Answer from the drawing. Dimensions are ordinates in mm from the lowest x, y and z of the part. A direction names the side the tool comes from. Coordinates: 2 decimals unless noted, no trailing zeros. Loops run counter-clockwise (first coordinate to the right, second up) from the corner with the lowest first, then second, coordinate; pieces in that order, holes last. Notation, with made-up numbers: (33.25, 54.25) - (88.25, 54.25) arc R15 cw to (88.25, 74.25) - close; hole circle Ø3 at (79, 74.25). An arc over 180 degrees is marked (long way). Use one line per item in the form item = value. Start each with the question number.
1) A cutting plane is placed at C-C (y = 8). Give the vertices of the cut face in (x, z), and give its area (3 significant figures).
2) Which of the six approach directions +Z, -Z, +X, -X, +Y, -Y give full straight-line access (tool end or side, diameter ignored) to the marked faces 1, 2 and 3?
3) Consider line 1 (X direction, y = 19, z = 37.4); line 2 (Y direction, x = 6.5, z = 43.75); line 3 (Y direction, x = 7, z = 28). Determine where each line is inside the solid, lowest interval first.
4) A cutting plane is placed at A-A (x = 14.5). Give the vertices of the cut face in (y, z), and give its area (3 significant figures).
5) A cutting plane is placed at D-D (z = 4.5). Give the vertices of the cut face in (x, y).
6) A cutting plane is placed at B-B (y = 19). Give the vertices of the cut face in (x, z), and give its area (3 significant figures).
7) Each of these flat-tipped pins is pushed along its axis until it touches: P1, Ø5, axis at x = 13.5, y = 20, coming from the -Z side; P2, Ø12.5, axis at x = 27.5, z = 39, coming from the -Y side; P3, Ø5, axis at x = 31.5, y = 19, coming from the -Z side; P4, Ø2, axis at x = 6.5, y = 19, coming from the -Z side. Where does it stop, or does it pass through?
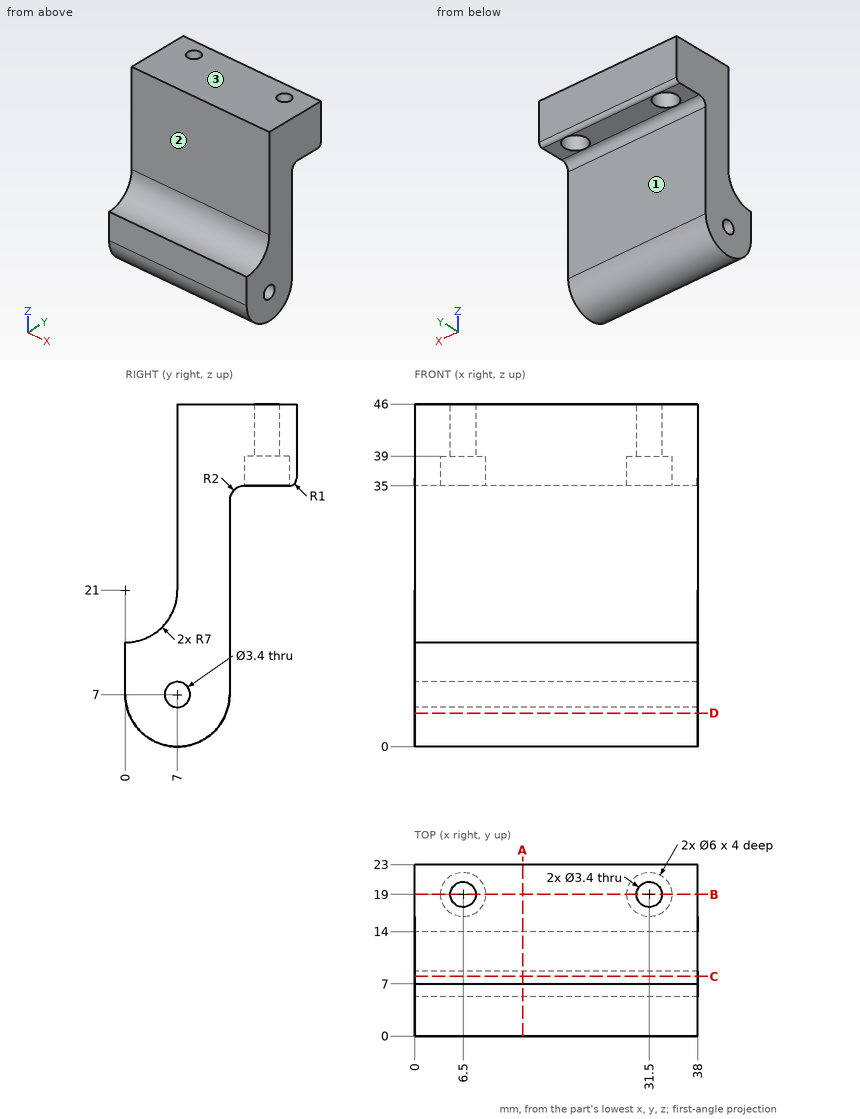
Found:
q1.outline = (0, 0.07) - (38, 0.07) - (38, 5.63) - (0, 5.63) - close; (0, 8.37) - (38, 8.37) - (38, 46) - (0, 46) - close
q1.area = 1,640 mm^2
q2.face_1 = -Z, +X, -X, +Y
q2.face_2 = +Z, +X, -X, -Y
q2.face_3 = +Z, +X, -X, +Y, -Y
q3.line_1 = 0 to 3.5, 9.5 to 28.5, 34.5 to 38
q3.line_2 = 7 to 17.3, 20.7 to 23
q3.line_3 = 7 to 14
q4.outline = (0, 7) arc R7 ccw to (14, 7) - (14, 33) arc R2 cw to (16, 35) - (22, 35) arc R1 ccw to (23, 36) - (23, 46) - (7, 46) - (7, 21) arc R7 cw to (0, 14) - close; hole circle Ø3.4 at (7, 7)
q4.area = 500 mm^2
q5.outline = (0, 0.46) - (38, 0.46) - (38, 13.54) - (0, 13.54) - close
q6.outline = (0, 35) - (3.5, 35) - (3.5, 39) - (4.8, 39) - (4.8, 46) - (0, 46) - close; (8.2, 39) - (9.5, 39) - (9.5, 35) - (28.5, 35) - (28.5, 39) - (29.8, 39) - (29.8, 46) - (8.2, 46) - close; (33.2, 39) - (34.5, 39) - (34.5, 35) - (38, 35) - (38, 46) - (33.2, 46) - close
q6.area = 322 mm^2
q7.P1 = 35
q7.P2 = 7
q7.P3 = 39
q7.P4 = through
